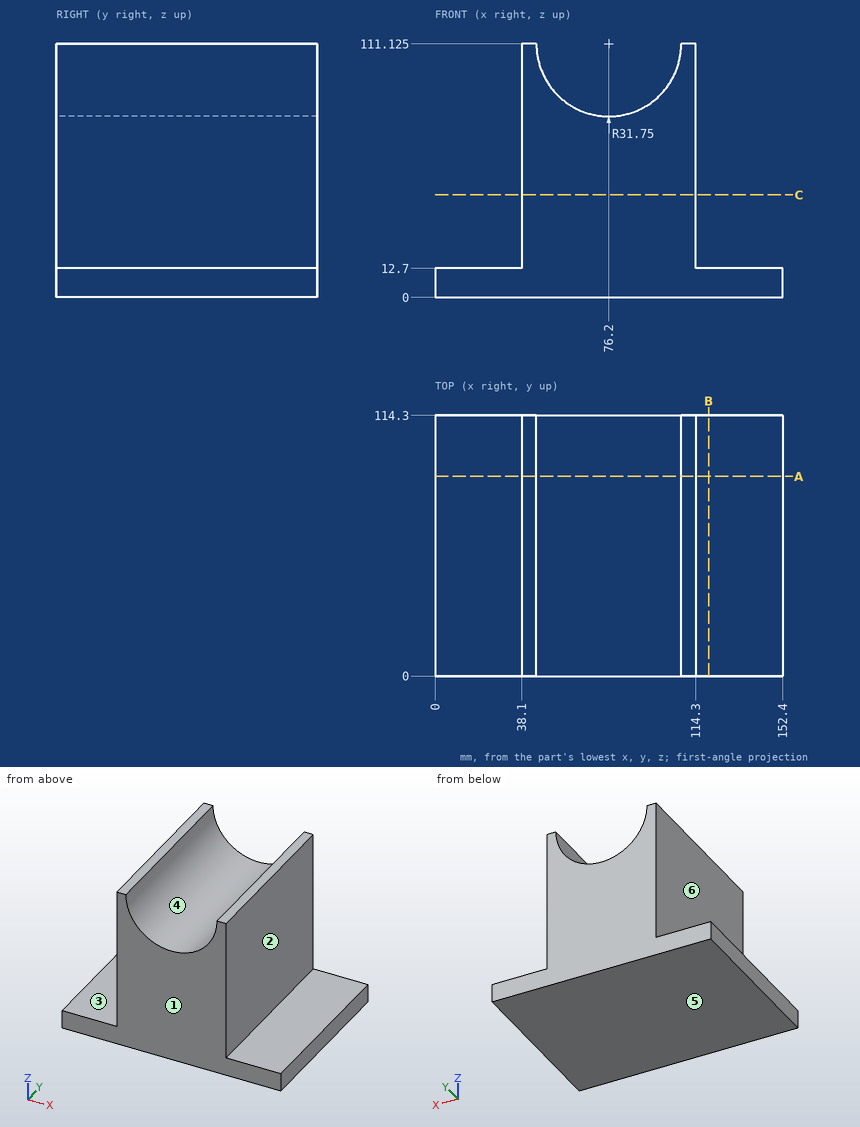
Design review of the part shown in the three views and the two pictorial views. Dimensions are in mm from the part's minimum x, y and z. A direction names the side the tool comes from. Round coordinates to 2 decimals unless told otherwise and drop trailing zeros. Write each loop counter-clockwise with the first axis right and the second up, starting at its lowest first coordinate (ties: lowest second). Pieces come first, ordered by that corner, then holes. Notation, with made-up numbers: (-20.5, 68) - (-2.5, 68) arc R24 cw to (-2.5, 100) - close; hole circle Ø8 at (76.25, 19.25). An arc over 180 degrees is marked (long way). Return JSON: item names as keys, results as strings. Group by question number.
Item 1: We need section B-B on x = 120. Write out the cut boundary in (y, z).
Item 2: We need section A-A on y = 87.5. Write out the cut boundary in (x, z) (3 decimals).
Item 3: The part is to be moulded in two halves that separate along X. For the marked faces 4, 5 and 6, say which applies: pulls with the +X half, pulls with the -X half, needs draft (parallel to the pull), parting line crosses it, or undercut.
Item 4: We need section C-C on z = 45. Write out the cut boundary in (x, y), and give its area (3 significant figures).
Item 5: For probe 1 along X at (y, z) = (40, 16); probe 2 along Z at (x, y) = (125.5, 107); probe 3 along X at (y, z) = (67, 83.5), list the stretches that pass through material, from the lowest coordinate up. Write a range as [from, to].
Item 6: Insertion check: P1, Ø8, axis at y = 72.5, z = 77.5, coming from the -X side; P2, Ø2, axis at x = 63.5, y = 56.5, coming from the +Z side; P3, Ø6, axis at y = 20.5, z = 21.5, coming from the +X side. Each pin has a flat end and moves straight along its axis. Give the tip position at first contact, or say it passes through.
Item 7: Machinability: for the marked faces 1, 2 and 3, which of the approach directions +Z, -Z, +X, -X, +Y, -Y give a long, thin tool a straight path to every point of the face, cutting with its end or side? Answer none if there is none.
Model answer:
{
 "1": {"outline": "(0, 0) - (114.3, 0) - (114.3, 12.7) - (0, 12.7) - close"},
 "2": {"outline": "(0, 0) - (152.4, 0) - (152.4, 12.7) - (114.3, 12.7) - (114.3, 111.125) - (107.95, 111.125) arc R31.75 cw to (44.45, 111.125) - (38.1, 111.125) - (38.1, 12.7) - (0, 12.7) - close"},
 "3": {"face 4": "undercut", "face 5": "needs draft", "face 6": "pulls with the -X half"},
 "4": {"outline": "(38.1, 0) - (114.3, 0) - (114.3, 114.3) - (38.1, 114.3) - close", "area": "8,710 mm²"},
 "5": {"probe 1": "x = [38.1, 114.3]", "probe 2": "z = [0, 12.7]", "probe 3": "x = [38.1, 60.55], [91.85, 114.3]"},
 "6": {"P1": "stops at x = 38.1", "P2": "stops at z = 82.48", "P3": "stops at x = 114.3"},
 "7": {"face 1": "+Z, -Z, +X, -X, -Y", "face 2": "+Z, +X, +Y, -Y", "face 3": "+Z, -X, +Y, -Y"}
}
